Source: three-view drawing plus pictorial views. Frame: mm from the lowest corner of the part. Give positions to 0.01 mm unless a question says otherwise; leave off trailing zeros. Loops run counter-clockwise (first coordinate to the right, second up) from the corner with the lowest first, then second, coordinate; pieces in that order, holes last.
1. Section C-C, the plane x = 53. Output: boundary loops of the cut face in (y, z).
2. Material intervals for line 1 along X through (y, z) = (0.75, 43.08) (1 decimal); line 2 along Z through (x, y) = (67, 2.35); line 3 along X through (y, z) = (2.45, 9) (1 decimal), sorted ascending.
3. Section B-B, the plane z = 25.4. Output: boundary loops of the cut face in (x, y) (1 decimal), then the cut area to 3 significant figures.
4. Section D-D, the plane y = 2.4. Output: boundary loops of the cut face in (x, z) (1 decimal).
5. Section A-A, the plane z = 43.08. Output: boundary loops of the cut face in (x, y) (1 decimal), then the cut area to 3 significant figures.
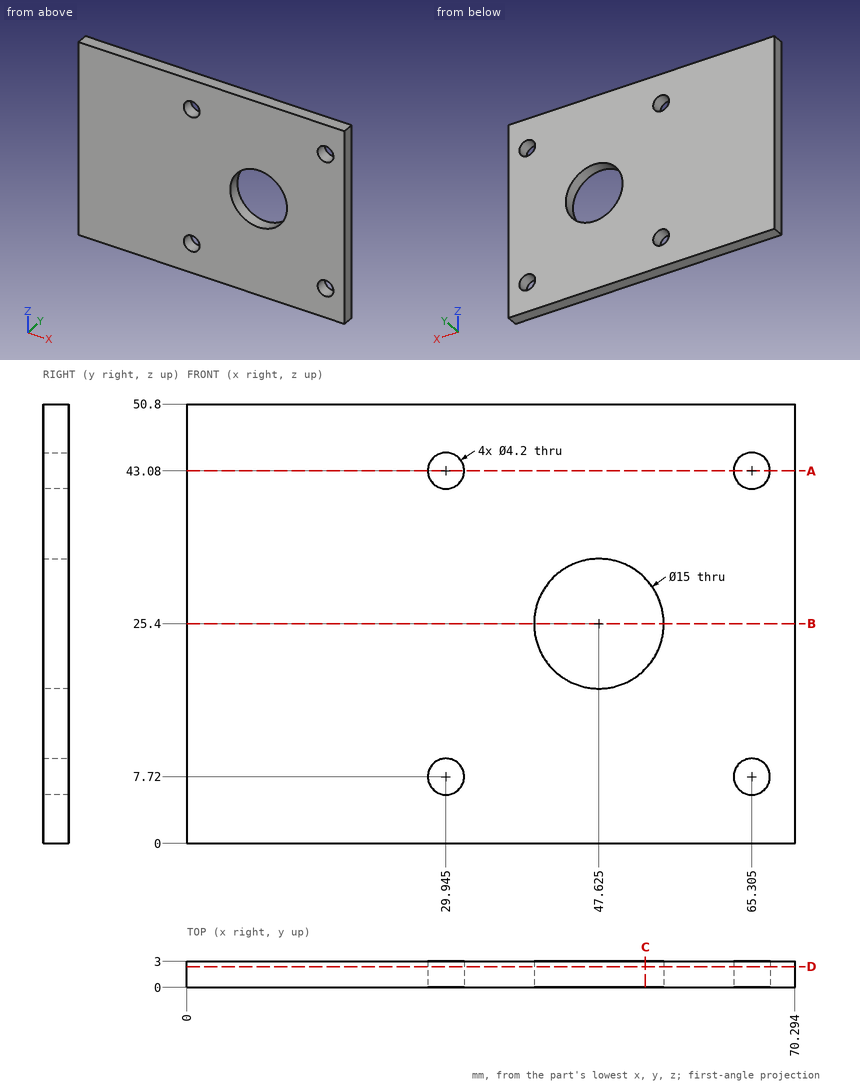
Answers below:
1. outline: (0, 0) - (3, 0) - (3, 20.17) - (0, 20.17) - close; (0, 30.63) - (3, 30.63) - (3, 50.8) - (0, 50.8) - close
2. line 1: x = 0 to 27.8, 32 to 63.2, 67.4 to 70.3
2. line 2: z = 0 to 6.48, 8.96 to 41.84, 44.32 to 50.8
2. line 3: x = 0 to 28.3, 31.6 to 63.6, 67 to 70.3
3. outline: (0, 0) - (40.1, 0) - (40.1, 3) - (0, 3) - close; (55.1, 0) - (70.3, 0) - (70.3, 3) - (55.1, 3) - close
3. area: 166 mm2
4. outline: (0, 0) - (70.3, 0) - (70.3, 50.8) - (0, 50.8) - close; hole circle Ø4.2 at (29.9, 7.7); hole circle Ø4.2 at (29.9, 43.1); hole circle Ø15 at (47.6, 25.4); hole circle Ø4.2 at (65.3, 7.7); hole circle Ø4.2 at (65.3, 43.1)
5. outline: (0, 0) - (27.8, 0) - (27.8, 3) - (0, 3) - close; (32, 0) - (63.2, 0) - (63.2, 3) - (32, 3) - close; (67.4, 0) - (70.3, 0) - (70.3, 3) - (67.4, 3) - close
5. area: 186 mm2
